from build123d import *

# Parameters (mm, degrees)
ESQUISSE1_R             = 6.5
BOSS_EXTRU_1_DEPTH      = 8
CONG_1_R                = 0.5
ENL_V_MAT_EXTRU_1_DEPTH = 4
CONG_2_R                = 0.5
ESQUISSE3_R             = 4
BOSS_EXTRU_2_DEPTH      = 35
CHANFREIN1_SIZE         = 0.2


with BuildPart() as part:
    # Esquisse1 → Boss.-Extru.1 (new body)
    with BuildSketch(Plane(origin=(0, 0, 0), x_dir=(0, 0, -1), z_dir=(1, 0, 0))):
        Circle(ESQUISSE1_R)
    extrude(amount=BOSS_EXTRU_1_DEPTH)

    # Congé1
    cong_1_edges = [part.edges().sort_by_distance(p)[0] for p in [
        (8, 0, 6.5),
    ]]
    fillet(cong_1_edges, radius=CONG_1_R)

    # Esquisse2 → Enlèv. mat.-Extru.1 (cut)
    with BuildSketch(Plane(origin=(8, 0, 0), x_dir=(0, 0, -1), z_dir=(1, 0, 0))):
        Polygon((1.732050808, -3), (3.464101615, 0), (1.732050808, 3), (-1.732050808, 3), (-3.464101615, 0), (-1.732050808, -3), align=None)
    extrude(amount=-ENL_V_MAT_EXTRU_1_DEPTH, mode=Mode.SUBTRACT)

    # Congé2
    cong_2_edges = [part.edges().sort_by_distance(p)[0] for p in [
        (4, -3, 0),
        (4, -1.5, 2.598076211),
        (4, 1.5, 2.598076211),
        (4, 3, 0),
        (4, 1.5, -2.598076211),
        (4, -1.5, -2.598076211),
    ]]
    fillet(cong_2_edges, radius=CONG_2_R)

    # Esquisse3 → Boss.-Extru.2 (add)
    with BuildSketch(Plane.ZY):
        with Locations(Location((0, 0, 0), (0, 0, 180))):  # turned: the seam where the file's is
            Circle(ESQUISSE3_R)
    extrude(amount=BOSS_EXTRU_2_DEPTH)

    # Esquisse4 → Enlèvement de matière-Révolution1 (revolve, cut)
    with BuildSketch(Plane(origin=(0, 0, 0), x_dir=(1, 0, 0), z_dir=(0, 1, 0))):
        Polygon((-7.046630766, 4), (-7, 3.9), (-6.953369234, 4), align=None)
    revolve(axis=Axis((-35, 0, 0), (1, 0, 0)), mode=Mode.SUBTRACT)

    # Chanfrein1
    chanfrein1_edges = [part.edges().sort_by_distance(p)[0] for p in [
        (-35, 0, 4),
    ]]
    chamfer(chanfrein1_edges, length=CHANFREIN1_SIZE)


solid = part.part
Can you work these out from the model? Positions are in its coordinate system, mm. A direction names the side the tool comes from. Coordinates: 2 decimals unless noted, no trailing zeros. Loops run counter-clockwise (first coordinate to the right, second up) from the corner with the lowest first, then second, coordinate; pieces in that order, holes last. Notation, with made-up numbers: (13, 74) - (63, 74) arc R22 ccw to (63, 97) - close; hole circle Ø9 at (-38.75, 58.25). An arc over 180 degrees is marked (long way). Answer as a JSON object with one key per item and string values. Group by question number.
Item 1: On a 3-axis mill with a long thin cutter (end or side, diameter ignored), from which of +Z, -Z, +X, -X, +Y, -Y can I reach the whole of each face in a straight line? I mean faces 1 (the face through (-35, 0, 0)), 2 (the face through (-3.428, 3.905, 0.867)), 3 (the face through (6, -3, 0)). Say none if no direction works.
Item 2: If we section it at C-C (x = -28.5): List the corners of the cut face in (y, z) for me, plus the area to 3 significant figures.
Item 3: If I drill on L1, parallel to Y at x = 4.5, z = 0; L2, parallel to X at y = 4.75, z = 3; L3, parallel to X at y = -0.25, z = -1, over which ranges is the centre line in solid material (lowest first)? Write a range as from..to.
Item 4: If we section it at B-B (z = 0): List the corners of the cut face in (x, y) for me.
Item 5: For pin 1 (1.5 mm diameter, centred on y = 1, z = -1, fed in from +X); pin 2 (5 mm diameter, centred on x = -14.5, y = 2, fed in from +Z), each with a flat end and sliding along its axis, tell me the tip position at first contact or that it passes through.
Item 6: If we section it at A-A (x = 5): List the corners of the cut face in (y, z) for me, plus the area to 3 significant figures.
Item 7: If we mould it in two halves opening along Z, with no side actions, what happens to faces 4 (the face through (8, -3, -3)), 5 (the face through (-20.729, 3.905, 0.867)), 6 (the face through (6.3, -1.5, -2.6))? For each: released by +Z, released by -Z, zero draft, split by the parting line, or undercut.
Returned:
{
 "1": {"face 1": "+Z, -Z, -X, +Y, -Y", "face 2": "-X", "face 3": "+X"},
 "2": {"outline": "circle Ø8 at (0, 0)", "area": "50.3 mm²"},
 "3": {"L1": "y = -6.5..-3, 3..6.5", "L2": "x = 0..8", "L3": "x = -35..4"},
 "4": {"outline": "(-35, -3.8) - (-34.8, -4) - (-7.05, -4) - (-7, -3.9) - (-6.95, -4) - (0, -4) - (0, -6.5) - (7.5, -6.5) arc R0.5 ccw to (8, -6) - (8, -3) - (4.5, -3) arc R0.5 cw to (4, -2.5) - (4, 2.5) arc R0.5 cw to (4.5, 3) - (8, 3) - (8, 6) arc R0.5 ccw to (7.5, 6.5) - (0, 6.5) - (0, 4) - (-6.95, 4) - (-7, 3.9) - (-7.05, 4) - (-34.8, 4) - (-35, 3.8) - close"},
 "5": {"pin 1": "stops at x = 4", "pin 2": "stops at z = 4"},
 "6": {"outline": "circle Ø13 at (0, 0); hole (-3, -1.73) - (0, -3.46) - (3, -1.73) - (3, 1.73) - (0, 3.46) - (-3, 1.73) - close", "area": "102 mm²"},
 "7": {"face 4": "zero draft", "face 5": "split by the parting line", "face 6": "undercut"}
}
